Here's the drawing with two shaded views (mm, measured from the low corner). I have some questions. A direction names the side the tool comes from. Give positions to 0.01 mm unless a question says otherwise; leave off trailing zeros. Write each loop counter-clockwise with the first axis right and the second up, starting at its lowest first coordinate (ties: lowest second). Pieces come first, ordered by that corner, then holes. Notation, with made-up numbers: (-12, 63) - (6, 63) arc R17 ccw to (6, 94) - close; hole circle Ø8 at (4, -12). An arc over 180 degrees is marked (long way). Answer as a JSON object with one key per item and string values. Group by question number.
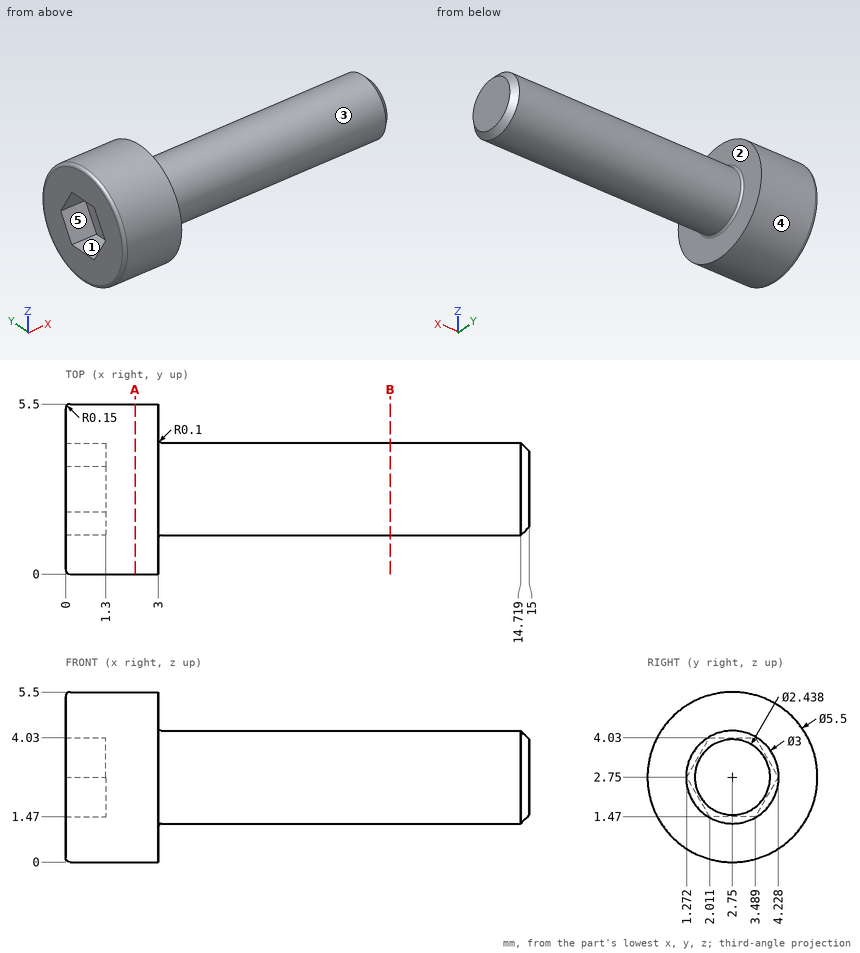
(1) I want a section at B-B, the plane x = 10.5. Please give me the cut outline in (y, z), and give its area (3 significant figures).
(2) If we mould it in two halves opening along Z, with no side actions, what happens to the marked faces 1, 2 and 3? For each: +Z half, -Z half, draft (parallel to the pull), parting line (faces both ways), or undercut.
(3) I need wall thicknesses on L1, parallel to Y at x = 7.75, z = 2.5; L2, parallel to X at y = 1.3, z = 4.05; L3, parallel to X at y = 1.9, z = 3.2. Which ranges of each line are inside material? Lowest first, please.
(4) Will this pin go through, and if not, where does the flat tip stop? P1, Ø1, axis at y = 1.5, z = 4.5, coming from the +X side.
(5) I want a section at A-A, the plane x = 2.25. Please give me the cut outline in (y, z), and give its area (3 significant figures).
(6) For the marked faces 4 and 5, which set-ups out of +Z, -Z, +X, -X, +Y, -Y let a thin tool reach every point of the face, with its end or its side?
Entries:
{
 "1": {"outline": "circle Ø3 at (2.75, 2.75)", "area": "7.07 mm^2"},
 "2": {"face 1": "undercut", "face 2": "draft", "face 3": "parting line"},
 "3": {"L1": "1.27 to 4.23", "L2": "0 to 3", "L3": "1.3 to 15"},
 "4": {"P1": "x = 3"},
 "5": {"outline": "circle Ø5.5 at (2.75, 2.75)", "area": "23.8 mm^2"},
 "6": {"face 4": "+X, -X", "face 5": "-X"}
}
